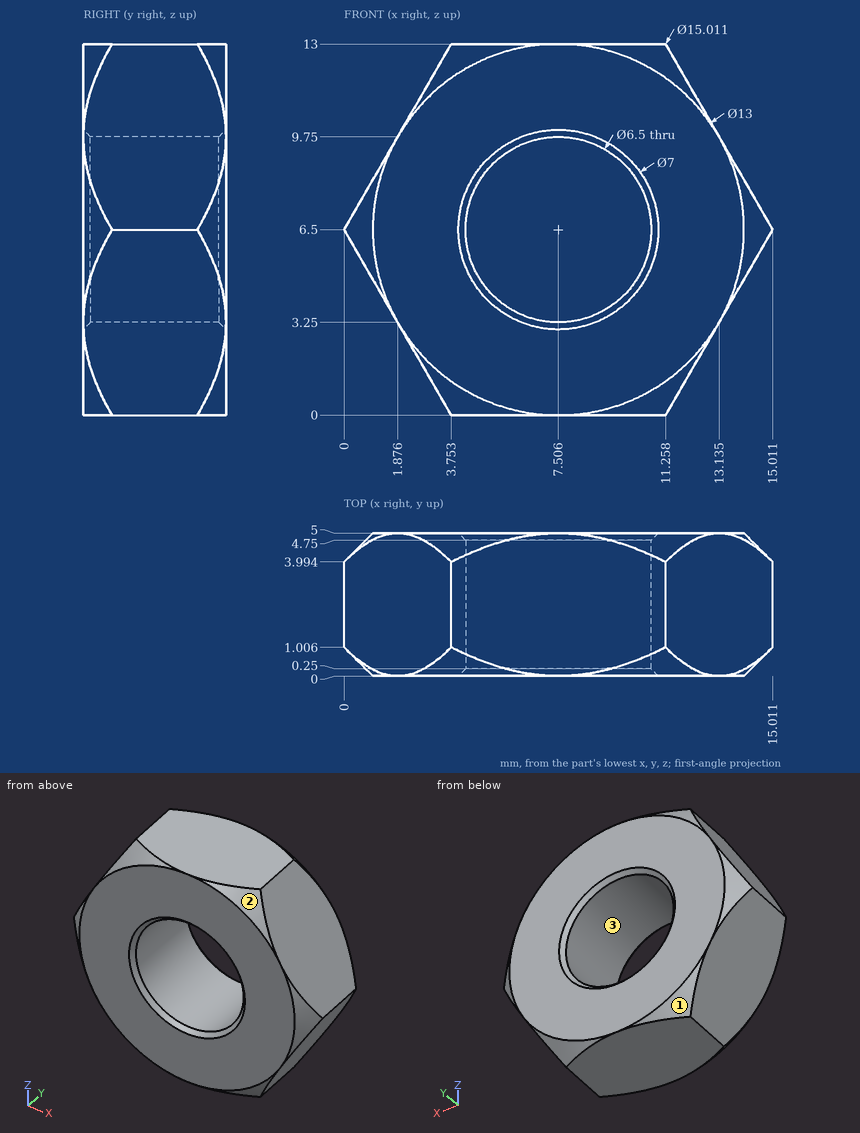
Check sheet for the drawn part. Datum: minimum x, y, z corner. Units: mm. Round coordinates to 2 decimals unless told otherwise and drop trailing zeros. Return JSON: item names as keys, results as strings.
Q1. Scan lines: L1, parallel to Z at x = 7.5, y = 3.6; L2, parallel to Z at x = 8.5, y = 2.15 (1 decimal); L3, parallel to X at y = 3.25, z = 9 (1 decimal). Record each from-to range of solid material in increasing order. Write a range as from..to.
Returned:
{"L1": "z = 0..3.25, 9.75..13", "L2": "z = 0..3.4, 9.6..13", "L3": "x = 1.4..5.4, 9.6..13.6"}
Q2. Draft check along X on the marked faces 1, 2 and 3. Enter one of: released by +X, released by -X, zero draft, split by the parting line, or undercut.
Returned:
{"face 1": "released by -X", "face 2": "released by +X", "face 3": "undercut"}
Q3. Depth check by flat-ended pin: P1, Ø1.5, axis at x = 8, z = 9, coming from the -Y side. Enter the tip coordinate at first touch or a pass-through.
Returned:
{"P1": "stops at y = 0.2"}
